from build123d import *

# Parameters (mm, degrees)
IZIM1_R                     = 1.6
Y_KSEKLIK_EKSTR_ZYON1_DEPTH = 4
IZIM2_R                     = 5.5
IZIM2_R_2                   = 1.6
Y_KSEKLIK_EKSTR_ZYON2_DEPTH = 3


with BuildPart() as part:
    # Çizim1 → Yükseklik-Ekstrüzyon1 (new body)
    with BuildSketch(Plane.XY):
        with BuildLine():
            ThreePointArc((-5.273709113, -1.561407118), (3.018112795, -4.597933792), (3.530207231, 4.2175392))
            ThreePointArc((3.530207231, 4.2175392), (2, 17.25), (3.530207231, 30.2824608))
            ThreePointArc((3.530207231, 30.2824608), (3.018112795, 39.097933792), (-5.273709113, 36.061407118))
            ThreePointArc((-5.273709113, 36.061407118), (-8, 17.25), (-5.273709113, -1.561407118))
        make_face()
        with Locations((0, 34.5)):
            Circle(IZIM1_R, mode=Mode.SUBTRACT)
        Circle(IZIM1_R, mode=Mode.SUBTRACT)
    extrude(amount=Y_KSEKLIK_EKSTR_ZYON1_DEPTH)

    # Çizim2 → Yükseklik-Ekstrüzyon2 (add)
    with BuildSketch(Plane.XY.offset(4)):
        with Locations(Location((0, 0, 0), (0, 0, 196.492641629))):
            Circle(IZIM2_R)
        Circle(IZIM2_R_2, mode=Mode.SUBTRACT)
    extrude(amount=Y_KSEKLIK_EKSTR_ZYON2_DEPTH)


solid = part.part
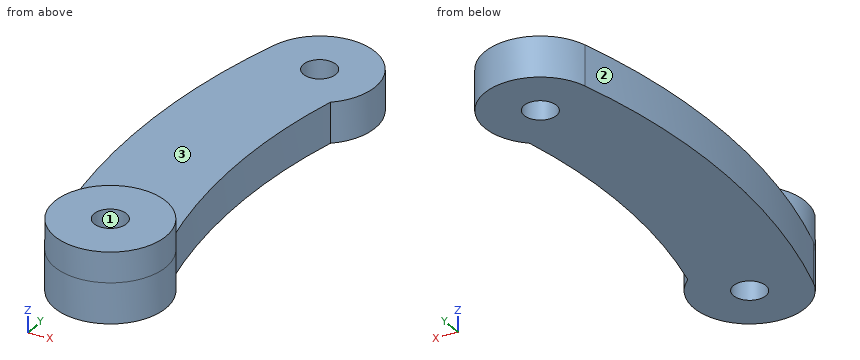
Design review of the part built by this model. Coordinates are the model's own, in mm. Face numbers are marked on the shaded views. Round coordinates to 2 decimals unless told otherwise and drop trailing zeros. Write each loop counter-clockwise with the first axis right and the second up, starting at its lowest first coordinate (ties: lowest second). Pieces come first, ordered by that corner, then holes. Notation, with made-up numbers: (29, -31) -> (49, -31) arc R21 ccw to (49, -25) -> close; hole circle Ø5 at (-13, 21.5). An arc over 180 degrees is marked (long way). One line per question, with ' | ' between items.
(1) Take a section at B-B, the plane y = 35. State the section outline as (x, z) points.
Result sheet:
outline: (-5.58, 0) -> (-1.52, 0) -> (-1.52, 4) -> (-5.58, 4) -> close; (1.52, 0) -> (5.48, 0) -> (5.48, 4) -> (1.52, 4) -> close
(2) Insertion check: P1, Ø8, axis at x = -6, y = 28.5, coming from the +Z side; P2, Ø4, axis at y = 24.5, z = 3, coming from the +X side; P3, Ø2.5, axis at x = 0, y = 0, coming from the -Z side. Each pin has a flat end and moves straight along its axis. Give the tip position at first contact, or say it passes through.
Result sheet:
P1: z = 4 | P2: x = 2.77 | P3: through
(3) Take a section at C-C, the plane z = 0.75. State how many separate pieces and enclosed holes the cut face has, and give its area (3 significant figures).
Result sheet:
separate pieces: 1 | enclosed holes: 2 | area: 436 mm2
(4) Wall thickness on line 1 (Y direction, x = 0, z = 3.5); line 2 (Y direction, x = 0, z = 4.75); line 3 (Y direction, x = -1.25, z = 0.75): over which ranges is each line inside the solid? List them lowest first. Write a range as [from, to].
Result sheet:
line 1: [-5.5, -1.6], [1.6, 32.9], [36.1, 40] | line 2: [-5.5, -1.6], [1.6, 5.5] | line 3: [-5.36, -1], [1, 33.5], [35.5, 39.86]
(5) Take a section at D-D, the plane x = 2.5. State the section outline as (y, z) points, and give its area (3 significant figures).
Result sheet:
outline: (-4.9, 0) -> (9.77, 0) -> (9.77, 4) -> (4.9, 4) -> (4.9, 7) -> (-4.9, 7) -> close; (24.73, 0) -> (39.4, 0) -> (39.4, 4) -> (24.73, 4) -> close | area: 147 mm2
(6) Take a section at A-A, the plane x = 0. State the section outline as (y, z) points.
Result sheet:
outline: (-5.5, 0) -> (-1.6, 0) -> (-1.6, 7) -> (-5.5, 7) -> close; (1.6, 0) -> (32.9, 0) -> (32.9, 4) -> (5.5, 4) -> (5.5, 7) -> (1.6, 7) -> close; (36.1, 0) -> (40, 0) -> (40, 4) -> (36.1, 4) -> close
(7) Draft analysis for pull direction X (two halves, no side actions). For the marked faces 1, 2 and 3, state which applies: released by +X, released by -X, zero draft, split by the parting line, or undercut.
Result sheet:
face 1: undercut | face 2: released by -X | face 3: zero draft
